CAD build for the part. Positions are in the model's coordinates, mm. Face numbers are marked on the shaded views. A direction names the side the tool comes from. Give positions to 0.01 mm unless a question says otherwise; leave off trailing zeros. Order: outer loops, then holes, each group sorted by start corner. A loop starts at its lowest first (then second) coordinate and runs counter-clockwise, first axis right, second up.
Item 1: Band-saw the part on A-A on y = -52. Give the cut face in (x, z).
Item 2: Which spindle directions (+Z, -Z, +X, -X, +Y, -Y) get a long thin tool onto all of the face, cutting with end or side? Do the marked faces 1 and 2. Say none if no direction does.
Item 3: Flat gauge pins, fed straight in: P1, Ø8, axis at y = -46, z = -10.5, coming from the -X side; P2, Ø5, axis at x = 66.5, z = -8, coming from the -Y side. Where does each tip first touch, or does it go through?
Item 4: Band-saw the part on B-B on z = -17. Give the cut face in (x, y).
Item 5: Wall check: L1, parallel to Z at x = 9.5, y = -42; L2, parallel to X at y = -54, z = -56; L3, parallel to Y at x = 13, z = -20.5. Give the ranges that are in metal, low to high.
Item 6: Two-plate mould, pull along X, no slides. Class the marked faces 3, 4 and 5: released by +X, released by -X, zero draft, split by the parting line, or undercut.
Item 7: Band-saw the part on C-C on x = 61.5. Give the cut face in (y, z), plus the area to 3 significant figures.
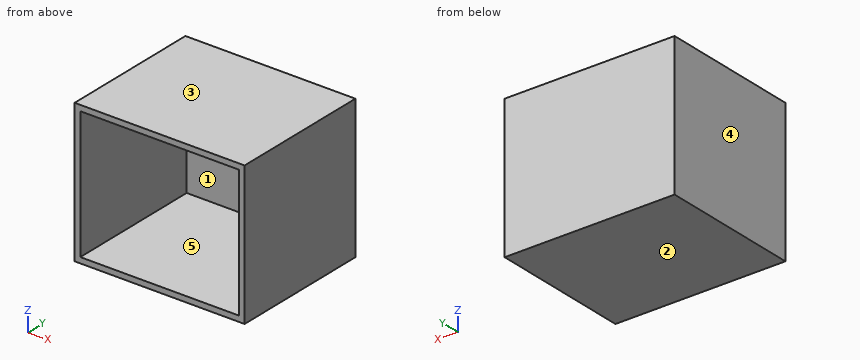
```python
from build123d import *

# Parameters (mm, degrees)
F0_W      = 12.7
F0_H      = 63.5
F1_DEPTH  = 63.5
F1_FACE_W = 63.5
F1_FACE_H = 63.5
F2_DEPTH  = 63.5
F3_T      = -2.54


with BuildPart() as f1:
    # F0 (on Front) → F1 (new body)
    with BuildSketch(Plane.XZ):
        with Locations((6.35, -31.75)):
            Rectangle(F0_W, F0_H)
    extrude(amount=F1_DEPTH)

    # F1_face (on face) → F2 (join)
    with BuildSketch(Plane(origin=(12.7, -31.75, -31.75), x_dir=(0, 1, 0), z_dir=(1, 0, 0))):
        Rectangle(F1_FACE_W, F1_FACE_H)
    extrude(amount=F2_DEPTH)

    # F3
    f3_openings = [f1.faces().sort_by_distance(p)[0] for p in [
        (38.1, -63.5, -31.75),
    ]]
    offset(amount=F3_T, openings=f3_openings)


solid = f1.part
```
The answers:
1. outline: (0, -63.5) - (76.2, -63.5) - (76.2, 0) - (0, 0) - close; hole (2.54, -60.96) - (73.66, -60.96) - (73.66, -2.54) - (2.54, -2.54) - close
2. face 1: -Y
2. face 2: -Z, +X, -X, +Y, -Y
3. P1: stops at x = 0
3. P2: stops at y = -2.54
4. outline: (0, -63.5) - (2.54, -63.5) - (2.54, -2.54) - (73.66, -2.54) - (73.66, -63.5) - (76.2, -63.5) - (76.2, 0) - (0, 0) - close
5. L1: z = -63.5 to -60.96, -2.54 to 0
5. L2: x = 0 to 2.54, 73.66 to 76.2
5. L3: y = -2.54 to 0
6. face 3: zero draft
6. face 4: released by -X
6. face 5: undercut
7. outline: (-63.5, -63.5) - (0, -63.5) - (0, 0) - (-63.5, 0) - (-63.5, -2.54) - (-2.54, -2.54) - (-2.54, -60.96) - (-63.5, -60.96) - close
7. area: 471 mm2
